from build123d import *

# Parameters (mm, degrees)
F0_W     = 15
F0_H     = 15
F1_DEPTH = 50
F2_W     = 15
F2_H     = 15
F3_DEPTH = 2
F5_DEPTH = 48.001


with BuildPart() as f1:
    # F0 (on Top) → F1 (new body)
    with BuildSketch(Plane.XY):
        with BuildLine():
            Line((-39.726279, 59.807934), (-43.190381, 57.807934))
            Line((-43.190381, 57.807934), (-12.990381, 5.5))
            Line((-12.990381, 5.5), (-25.980762, -2))
            ThreePointArc((-25.980762, -2), (-15, -12.980762), (0, -17))
            ThreePointArc((0, -17), (15, -12.980762), (25.980762, -2))
            Line((25.980762, -2), (12.990381, 5.5))
            Line((12.990381, 5.5), (43.190381, 57.807934))
            Line((43.190381, 57.807934), (39.726279, 59.807934))
            Line((39.726279, 59.807934), (30.599564, 44))
            Line((30.599564, 44), (0, 44))
            Line((0, 44), (-30.599564, 44))
            Line((-30.599564, 44), (-39.726279, 59.807934))
        make_face()
        Rectangle(F0_W, F0_H, mode=Mode.SUBTRACT)
        Polygon((-28.290163, 40), (28.290163, 40), (12.124356, 12), (-12.124356, 12), align=None, mode=Mode.SUBTRACT)
    extrude(amount=F1_DEPTH)

    # F2 (on Top) → F3 (join)
    with BuildSketch(Plane.XY):
        Rectangle(F2_W, F2_H)
    extrude(amount=F3_DEPTH)

    # F4 (on face) → F5 (cut, through all)
    with BuildSketch(Plane.XY.offset(2)):
        Polygon((7.5, 4.5), (7.5, -4.5), (8, -3.633975), (8, 3.633975), align=None)
        Polygon((-4.5, 7.5), (4.5, 7.5), (3.633975, 8), (-3.633975, 8), align=None)
        Polygon((-7.5, -4.5), (-7.5, 4.5), (-8, 3.633975), (-8, -3.633975), align=None)
        Polygon((4.5, -7.5), (-4.5, -7.5), (-3.633975, -8), (3.633975, -8), align=None)
    extrude(amount=F5_DEPTH, mode=Mode.SUBTRACT)


solid = f1.part
Design review of the part built by this model. Coordinates are the model's own, in mm. A direction names the side the tool comes from. Coordinates: 2 decimals unless noted, no trailing zeros. Order: outer loops, then holes, each group sorted by start corner. A loop starts at its lowest first (then second) coordinate and runs counter-clockwise, first axis right, second up. Notation, with made-up numbers: (38, -6.5) - (90, -6.5) arc R25 ccw to (90, 10.5) - close; hole circle Ø2 at (-1.5, 52.25). An arc over 180 degrees is marked (long way). Put each result on its own line as item: value.
1) Tool access review of faces 4 (the face through (19.577, 1.698, 24.65)), 5 (the face through (0, 44, 25)), 6 (the face through (20.32, 26.196, 24.65)), 7 (the face through (0, 10, 0)), 8 (the face through (0, -8, 26)): name each direction out of +Z, -Z, +X, -X, +Y, -Y from which nothing blocks a thin tool from reaching the whole face with its end or side.
Response values:
face 4: +Z, -Z, +X
face 5: +Z, -Z, +Y
face 6: +Z, -Z
face 7: -Z, +X, -X, +Y, -Y
face 8: +Z
2) Wall thickness on L1, parallel to X at y = 5.5, z = 27.5; L2, parallel to Y at x = 4, z = 31; L3, parallel to X at y = 39.5, z = 28: over which ranges is each line inside the solid? List them lowest first. Write a range as from..to.
Response values:
L1: x = -12.99..-7.5, 7.5..12.99
L2: y = -16.73..-7.79, 7.79..12, 40..44
L3: x = -32.62..-28, 28..32.62
3) The part is to be moulded in two halves that separate along Y. For faces 1 (the face through (0, 10, 50)), 2 (the face through (-7.5, -6, 26)), 3 (the face through (-35.099, 51.793, 24.65)), say which applies: released by +Y, released by -Y, zero draft, split by the parting line, or undercut.
Response values:
face 1: zero draft
face 2: undercut
face 3: released by +Y
4) Take a section at A-A, the plane x = -21. Give the boundary of the cut face in (y, z).
Response values:
outline: (-8.42, 0) - (0.88, 0) - (0.88, 50) - (-8.42, 50) - close; (19.37, 0) - (27.37, 0) - (27.37, 50) - (19.37, 50) - close; (40, 0) - (44, 0) - (44, 50) - (40, 50) - close
5) Take a section at D-D, the plane y = 2.5. Give the boundary of the cut face in (x, z), and give its area (3 significant figures).
Response values:
outline: (-18.19, 0) - (18.19, 0) - (18.19, 50) - (8, 50) - (8, 2) - (-8, 2) - (-8, 50) - (-18.19, 50) - close
area: 1,050 mm²
6) Take a section at C-C, the plane x = -2.5. Give the boundary of the cut face in (y, z), and give its area (3 significant figures).
Response values:
outline: (-16.9, 0) - (12, 0) - (12, 50) - (8, 50) - (8, 2) - (-8, 2) - (-8, 50) - (-16.9, 50) - close; (40, 0) - (44, 0) - (44, 50) - (40, 50) - close
area: 877 mm²
7) Take a section at B-B, the plane y = 19. Give the boundary of the cut face in (x, z), and give its area (3 significant figures).
Response values:
outline: (-20.78, 0) - (-16.17, 0) - (-16.17, 50) - (-20.78, 50) - close; (16.17, 0) - (20.78, 0) - (20.78, 50) - (16.17, 50) - close
area: 462 mm²
8) Insertion check: P1, Ø2.5, axis at x = 6, z = 24.5, coming from the -Y side; P2, Ø1.5, axis at y = -6, z = 27.5, coming from the -X side; P3, Ø8, axis at y = 1.5, z = 33.5, coming from the +X side. Each pin has a flat end and moves straight along its axis. Give the tip position at first contact, or say it passes through.
Response values:
P1: stops at y = -16.62
P2: stops at x = -23.81
P3: stops at x = 25.98
